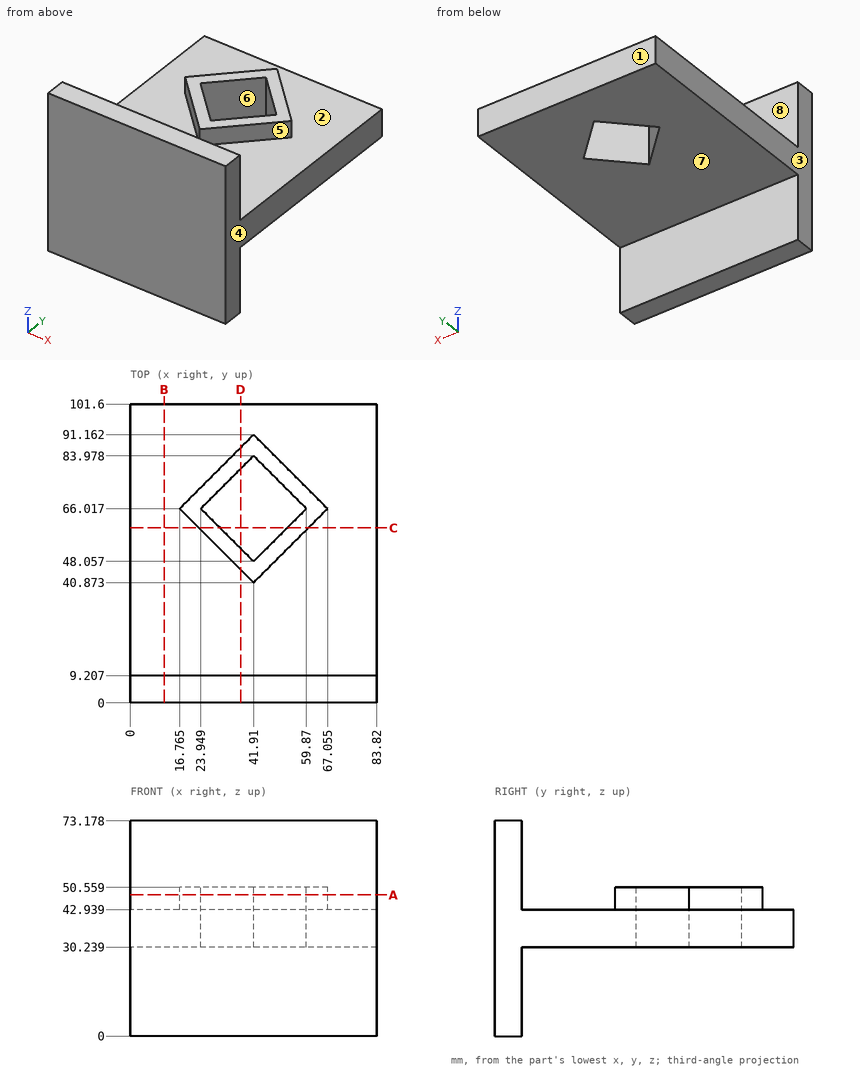
The figure shows three views and two pictorial views of one solid part (mm, origin at its lowest corner). Answer the questions. A direction names the side the tool comes from. Round coordinates to 2 decimals unless told otherwise and drop trailing zeros. Write each loop counter-clockwise with the first axis right and the second up, starting at its lowest first coordinate (ties: lowest second). Pieces come first, ordered by that corner, then holes. Notation, with made-up numbers: (4, 43.25) - (58, 43.25) arc R16 cw to (58, 48.25) - close; hole circle Ø3 at (-14.5, -33). An arc over 180 degrees is marked (long way). Use one line per item in the form item = value. Start each with the question number.
Item 1: A cutting plane is placed at A-A (z = 48). Give the number of separate pieces and of enclosed holes in the cut face, plus the area to 3 significant figures.
Item 2: A cutting plane is placed at B-B (x = 11.5). Write down the section's boundary in (y, z), plus the area to 3 significant figures.
Item 3: A cutting plane is placed at C-C (y = 59.5). Write down the section's boundary in (x, z).
Item 4: Flat-ended cylindrical pins translate along their axes: pin 1 Ø3 at (x, z) = (41.5, 27.5) entering from +Y; pin 2 Ø1 at (x, y) = (32.5, 57) entering from -Z; pin 3 Ø9 at (x, z) = (23.5, 51.5) entering from +Y. Find the tip coordinate at first contact, or state that the pin passes through.
Item 5: A tool of negligible diameter and unlimited length cuts with its end or side. For the marked faces 4, 5, 6, 7 and 8, from which of +Z, -Z, +X, -X, +Y, -Y can it reach the whole face along a straight path? Write none if from no direction.
Item 6: Determine the mould class of the marked faces 1, 2 and 3 for opening direction Y: +Y half, -Y half, draft (parallel to the pull), parting line (faces both ways), or undercut.
Item 7: A cutting plane is placed at D-D (x = 37.5). Write down the section's boundary in (y, z).
Item 8: Find the intervals of material crossed by line 1 (Y direction, x = 48.5, z = 47) (1 decimal); line 2 (Z direction, x = 73.5, y = 54.5); line 3 (Y direction, x = 13, z = 22.5), in increasing order. Write a range as [from, to].
The answers:
q1.separate_pieces = 2
q1.enclosed_holes = 1
q1.area = 1,390 mm^2
q2.outline = (0, 0) - (9.21, 0) - (9.21, 30.24) - (101.6, 30.24) - (101.6, 42.94) - (9.21, 42.94) - (9.21, 73.18) - (0, 73.18) - close
q2.area = 1,850 mm^2
q3.outline = (0, 30.24) - (30.47, 30.24) - (30.47, 50.56) - (23.28, 50.56) - (23.28, 42.94) - (0, 42.94) - close; (53.35, 30.24) - (83.82, 30.24) - (83.82, 42.94) - (60.54, 42.94) - (60.54, 50.56) - (53.35, 50.56) - close
q4.pin_1 = 9.21
q4.pin_2 = 30.24
q4.pin_3 = 77.15
q5.face_4 = +Z, -Z, +X, +Y, -Y
q5.face_5 = +Z, +X
q5.face_6 = +Z, -Z
q5.face_7 = -Z, +X, -X, +Y
q5.face_8 = +Z, +X, -X
q6.face_1 = +Y half
q6.face_2 = undercut
q6.face_3 = draft
q7.outline = (0, 0) - (9.21, 0) - (9.21, 30.24) - (52.47, 30.24) - (52.47, 50.56) - (45.28, 50.56) - (45.28, 42.94) - (9.21, 42.94) - (9.21, 73.18) - (0, 73.18) - close; (79.57, 30.24) - (101.6, 30.24) - (101.6, 42.94) - (86.75, 42.94) - (86.75, 50.56) - (79.57, 50.56) - close
q8.line_1 = [0, 9.2], [47.5, 54.6], [77.4, 84.6]
q8.line_2 = [30.24, 42.94]
q8.line_3 = [0, 9.21]
